```python
from build123d import *

# Parameters (mm, degrees)
EXTRUDE_1_DEPTH     = 2
SKETCH_2_W          = 12.24406528
SKETCH_2_H          = 8.971692278
CUT_EXTRUDE_1_DEPTH = 1
CHAMFER_1_SIZE      = 0.5
CHAMFER_1_SIZE2     = 2
CHAMFER_2_SIZE      = 2
CHAMFER_2_SIZE2     = 0.5
FILLET_1_R          = 0.1


with BuildPart() as part:
    # Эскиз1 → Бобышка-Вытянуть1 (new body)
    with BuildSketch(Plane(origin=(0, 0, 0), x_dir=(0, 0, -1), z_dir=(1, 0, 0))):
        with BuildLine():
            Line((0, 0), (0, 1.1))
            Line((0, 1.1), (2, 2))
            Line((2, 2), (14.5, 2))
            Line((14.5, 2), (14.5, 4))
            Line((14.5, 4), (20.3, 4))
            Line((20.3, 4), (19.722649731, 3))
            Line((19.722649731, 3), (20.8, 3))
            Line((20.8, 3), (20.8, 2.8))
            Line((20.8, 2.8), (25.5, 2.8))
            ThreePointArc((25.5, 2.8), (27.3, 1), (25.5, -0.8))
            Line((25.5, -0.8), (20.8, -0.8))
            Line((20.8, -0.8), (20.8, -1))
            Line((20.8, -1), (19.722649731, -1))
            Line((19.722649731, -1), (20.3, -2))
            Line((20.3, -2), (2, -2))
            Line((2, -2), (0, -1.1))
            Line((0, -1.1), (0, 0))
        make_face()
        with BuildLine():
            Line((23.5, 1.9), (25.5, 1.9))
            ThreePointArc((25.5, 1.9), (26.4, 1), (25.5, 0.1))
            Line((25.5, 0.1), (23.5, 0.1))
            ThreePointArc((23.5, 0.1), (22.6, 1), (23.5, 1.9))
        make_face(mode=Mode.SUBTRACT)
    extrude(amount=EXTRUDE_1_DEPTH)

    # Эскиз2 → Вырез-Вытянуть1 (cut)
    with BuildSketch(Plane(origin=(2, 0, 0), x_dir=(0, 0, -1), z_dir=(1, 0, 0))):
        with Locations((23.12203264, 1.144281601)):
            Rectangle(SKETCH_2_W, SKETCH_2_H)
    extrude(amount=-CUT_EXTRUDE_1_DEPTH, mode=Mode.SUBTRACT)

    # Фаска1
    chamfer_1_edges = [part.edges().sort_by_distance(p)[0] for p in [
        (2, 0, 0),
    ]]
    chamfer_1_side = [part.faces().sort_by_distance(p)[0] for p in [
        (1, 0, 0),
    ]]
    chamfer(chamfer_1_edges, length=CHAMFER_1_SIZE, length2=CHAMFER_1_SIZE2, reference=chamfer_1_side[0])

    # Фаска2
    chamfer_2_edges = [part.edges().sort_by_distance(p)[0] for p in [
        (0, 0, 0),
    ]]
    chamfer_2_side = [part.faces().sort_by_distance(p)[0] for p in [
        (0, 0.481010429, -13.197583299),
    ]]
    chamfer(chamfer_2_edges, length=CHAMFER_2_SIZE, length2=CHAMFER_2_SIZE2, reference=chamfer_2_side[0])

    # Скругление1
    fillet_1_edges = [part.edges().sort_by_distance(p)[0] for p in [
        (0, 2.8, -23.15),
        (0, 1, -27.3),
        (0, -0.8, -23.15),
        (0, 1, -22.6),
        (0, 0.1, -24.5),
        (0, 1, -26.4),
        (0, 1.9, -24.5),
        (1, 1.9, -24.5),
        (1, 1, -22.6),
        (1, 0.1, -24.5),
        (1, 1, -26.4),
        (1, -0.8, -23.15),
        (1, 1, -27.3),
        (1, 2.8, -23.15),
    ]]
    fillet(fillet_1_edges, radius=FILLET_1_R)


solid = part.part
```
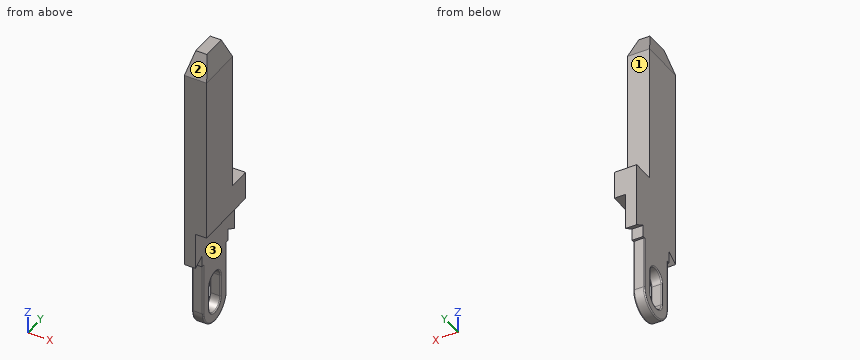
Read the model definition and answer for the solid it produces. Units are mm, in the model's axes. Face numbers are marked on the shaded views. A direction names the side the tool comes from. Coordinates: 2 decimals unless noted, no trailing zeros. Order: outer loops, then holes, each group sorted by start corner. A loop starts at its lowest first (then second) coordinate and runs counter-clockwise, first axis right, second up. Notation, with made-up numbers: (55, 13) - (100, 13) arc R20 cw to (100, 52) - close; hole circle Ø6 at (-23.75, 15). An arc over 180 degrees is marked (long way). Answer as a JSON object with one key per item and string values. Group by question number.
Item 1: Flat-ended cylindrical pins translate along their axes: P1, Ø0.9, axis at x = 0.5, z = -24, coming from the -Y side; P2, Ø1, axis at y = 1, z = -18, coming from the +X side; P3, Ø0.9, axis at x = 0.5, z = -24.5, coming from the +Y side. Find the tip coordinate at first contact, or state that the pin passes through.
Item 2: Section B-B (y = 3.6) is taken. Give the vertices of the cut face in (x, z), plus the area to 3 significant figures.
Item 3: A tool of negligible diameter and unlimited length cuts with its end or side. For the marked faces 1, 2 and 3, from which of +Z, -Z, +X, -X, +Y, -Y can it reach the whole face along a straight path? Write none if from no direction.
Item 4: Consider probe 1 along X at (y, z) = (0.3, -18); probe 2 along Y at (x, z) = (0.9, -3.25); probe 3 along Z at (x, y) = (1.35, 3.45). Determine where each line is inside the solid, lowest interval first. Write a range as from..to.
Item 5: Section A-A (z = -6.25) is taken. Give the vertices of the cut face in (x, y).
Results are:
{
 "1": {"P1": "stops at y = -0.8", "P2": "stops at x = 1", "P3": "stops at y = 2.8"},
 "2": {"outline": "(0, -20.07) - (1, -20.07) - (1, -17) - (2, -17) - (2, -14.5) - (0, -14.5) - close", "area": "8.07 mm^2"},
 "3": {"face 1": "+Z, +X, -X, +Y", "face 2": "+Z, +X, -X, -Y", "face 3": "-Z, +X, +Y, -Y"},
 "4": {"probe 1": "x = 0..1", "probe 2": "y = -2..2", "probe 3": "z = -17..-14.5"},
 "5": {"outline": "(0, -2) - (2, -2) - (2, 2) - (0, 2) - close"}
}
